Geometry: see drawing. Coordinates: mm, zero at the bounding-box minimum. A direction names the side the tool comes from. Round coordinates to 2 decimals unless told otherwise and drop trailing zeros. Write each loop counter-clockwise with the first axis right and the second up, starting at its lowest first coordinate (ties: lowest second). Pieces come first, ordered by that corner, then holes. Notation, with made-up numbers: (1.5, 12) -> (17.5, 12) arc R21 cw to (17.5, 47) -> close; hole circle Ø5 at (60, 68.5). An arc over 180 degrees is marked (long way). Use CSV: the item, a comma, the result in double quotes.
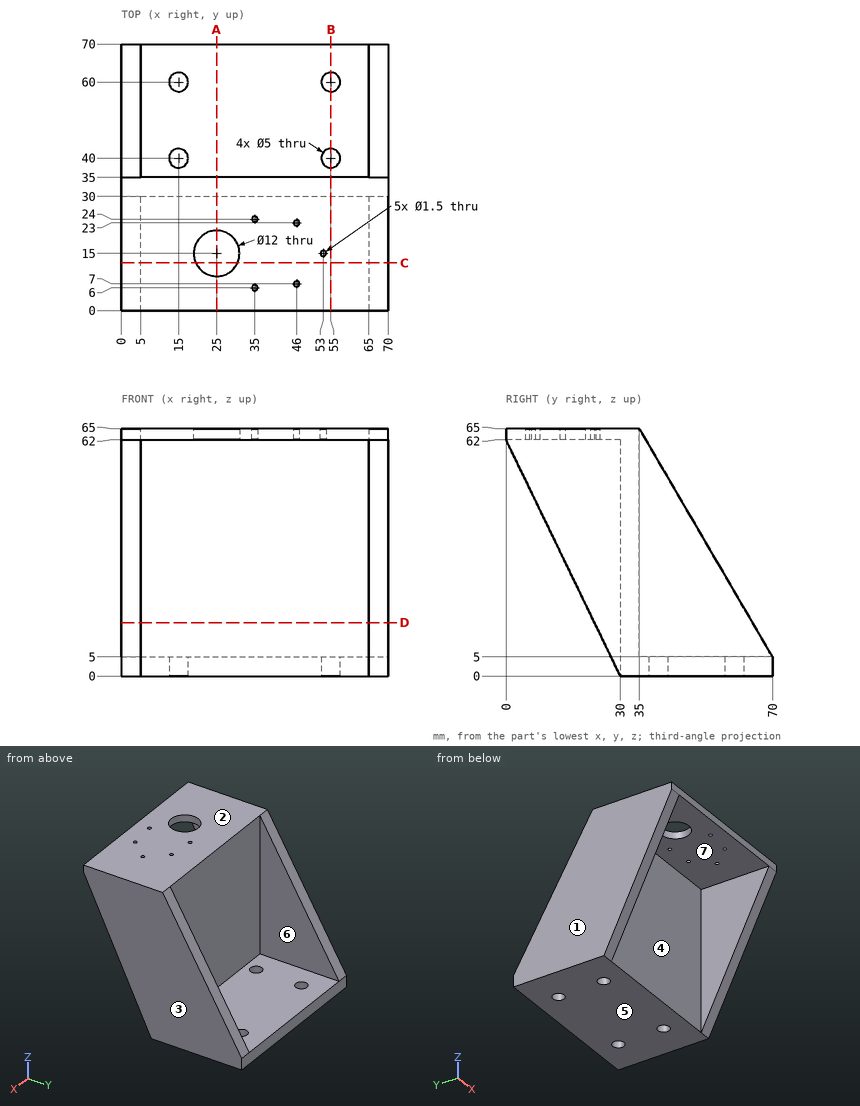
Item 1: Pull-direction query (X, two-part tool) for the marked faces 1, 2, 3 and 4; classes: +X half, -X half, draft (parallel to the pull), parting line (faces both ways), or undercut.
Worked answers:
face 1,"-X half"
face 2,"draft"
face 3,"+X half"
face 4,"undercut"
Item 2: Section query A-A on x = 25. Return the cut outline in (y, z).
Worked answers:
outline,"(0, 62) -> (9, 62) -> (9, 65) -> (0, 65) -> close; (21, 62) -> (30, 62) -> (30, 0) -> (70, 0) -> (70, 5) -> (35, 5) -> (35, 65) -> (21, 65) -> close"
Item 3: Set-up query: the marked faces 5, 6 and 7. Return all of +Z, -Z, +X, -X, +Y, -Y with unobstructed straight access to the full face (end or side cutting, diameter ignored); none if empty.
Worked answers:
face 5,"-Z, +X, -X, +Y, -Y"
face 6,"+Z, +Y"
face 7,"-Z, -Y"
Item 4: Section query D-D on z = 14. Return the cut outline in (x, y).
Worked answers:
outline,"(0, 23.23) -> (5, 23.23) -> (5, 30) -> (65, 30) -> (65, 23.23) -> (70, 23.23) -> (70, 64.75) -> (65, 64.75) -> (65, 35) -> (5, 35) -> (5, 64.75) -> (0, 64.75) -> close"
Item 5: Section query B-B on x = 55. Return the cut outline in (y, z), plus the area to 3 significant figures.
Worked answers:
outline,"(0, 62) -> (30, 62) -> (30, 0) -> (37.5, 0) -> (37.5, 5) -> (35, 5) -> (35, 65) -> (0, 65) -> close; (42.5, 0) -> (57.5, 0) -> (57.5, 5) -> (42.5, 5) -> close; (62.5, 0) -> (70, 0) -> (70, 5) -> (62.5, 5) -> close"
area,"540 mm²"
Item 6: Line query: line 1 (Y direction, x = 55, z = 3.35); line 2 (Y direction, x = 25, z = 64); line 3 (X direction, y = 49.5, z = 32). Output: solid intervals per line, ascending.
Worked answers:
line 1,"y = 30 to 37.5, 42.5 to 57.5, 62.5 to 70"
line 2,"y = 0 to 9, 21 to 35"
line 3,"x = 0 to 5, 65 to 70"
Item 7: Section query C-C on y = 12.5. Return the cut outline in (x, z).
Worked answers:
outline,"(0, 36.17) -> (5, 36.17) -> (5, 62) -> (19.55, 62) -> (19.55, 65) -> (0, 65) -> close; (30.45, 62) -> (65, 62) -> (65, 36.17) -> (70, 36.17) -> (70, 65) -> (30.45, 65) -> close"
Item 8: First-contact query: pin 1 Ø10 at (x, z) = (47.5, 24.5) entering from +Y; pin 2 Ø15 at (x, y) = (26.5, 12) entering from -Z; pin 3 Ø17.5 at (x, y) = (41, 58.5) entering from +Z; pin 4 Ø4 at (x, y) = (15, 40) entering from -Z. Flat tips, straight axial feed; report the tip coordinate or a pass-through.
Worked answers:
pin 1,"stops at y = 35"
pin 2,"stops at z = 62"
pin 3,"stops at z = 5"
pin 4,"passes through"
